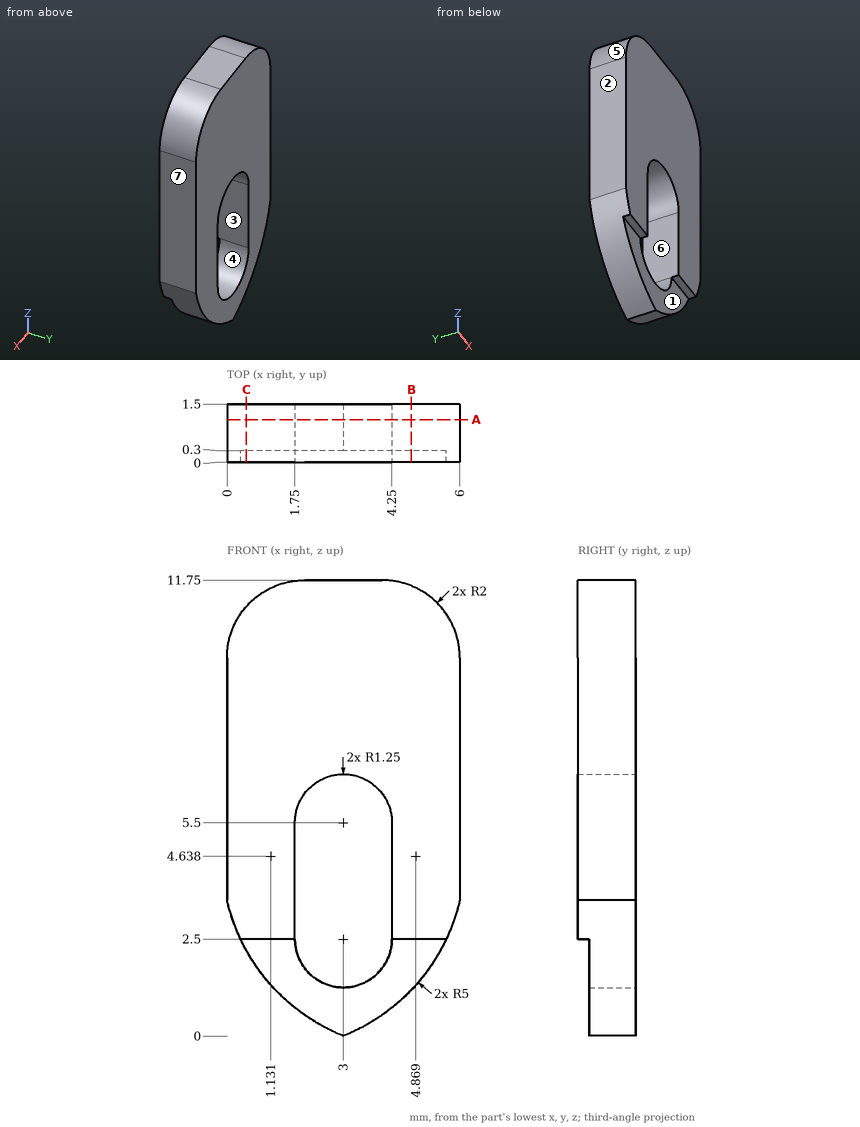
Study the drawing (mm; zero at the part's minimum x, y, z) and answer. A direction names the side the tool comes from. Give positions to 0.01 mm unless a question says otherwise; leave off trailing zeros. Order: outer loops, then holes, each group sorted by start corner. A loop starts at its lowest first (then second) coordinate and runs counter-clockwise, first axis right, second up. Notation, with made-up numbers: (48.25, -18.75) -> (65.25, -18.75) arc R30 cw to (65.25, 18.25) -> close; hole circle Ø11 at (80, 71). An arc over 180 degrees is marked (long way). Put each result on its own line as item: value.
Item 1: For a pull along Z with two mould halves and no side action, classify the marked faces 4, 5, 6 and 7 as released by +Z, released by -Z, zero draft, split by the parting line, or undercut.
Established:
face 4: undercut
face 5: released by +Z
face 6: undercut
face 7: zero draft
Item 2: Given P1, Ø0.8, axis at x = 3.5, z = 1, coming from the -Y side, flat-ended and moving along its own axis, determine where the tip first touches the part or whether it passes through.
Established:
P1: stops at y = 0.3
Item 3: A cutting plane is placed at B-B on x = 4.75. Give the vertices of the cut face in (y, z).
Established:
outline: (0, 2.5) -> (0.3, 2.5) -> (0.3, 1.19) -> (1.5, 1.19) -> (1.5, 11.6) -> (0, 11.6) -> close
Item 4: A cutting plane is placed at A-A on y = 1.1. Give the vertices of the cut face in (x, z).
Established:
outline: (0, 3.5) arc R5 ccw to (3, 0) arc R5 ccw to (6, 3.5) -> (6, 9.75) arc R2 ccw to (4, 11.75) -> (2, 11.75) arc R2 ccw to (0, 9.75) -> close; hole (1.75, 2.5) arc R1.25 ccw to (4.25, 2.5) -> (4.25, 5.5) arc R1.25 ccw to (1.75, 5.5) -> close
Item 5: A cutting plane is placed at C-C on x = 0.5. Give the vertices of the cut face in (y, z).
Established:
outline: (0, 2.5) -> (0.3, 2.5) -> (0.3, 2.21) -> (1.5, 2.21) -> (1.5, 11.07) -> (0, 11.07) -> close
Item 6: For the marked faces 1, 2 and 3, determine the directions among +Z, -Z, +X, -X, +Y, -Y from which every point of the face is accessible in a straight line to the end or side of a thin tool.
Established:
face 1: -Z, +X, -X, -Y
face 2: +Z, -Z, -X, +Y, -Y
face 3: +Y, -Y
Item 7: Straight lines are drawn through the part: line 1 (X direction, y = 0.75, z = 5.25); line 2 (Y direction, x = 1.75, z = 1); line 3 (X direction, y = 1.45, z = 2) (1 decimal). For each, find the intervals that lie inside material, in ascending order.
Established:
line 1: x = 0 to 1.75, 4.25 to 6
line 2: y = 0.3 to 1.5
line 3: x = 0.6 to 1.9, 4.1 to 5.4
